Design review of the part built by this model. Coordinates are the model's own, in mm. Give positions to 0.01 mm unless a question says otherwise; leave off trailing zeros. Loops run counter-clockwise (first coordinate to the right, second up) from the corner with the lowest first, then second, coordinate; pieces in that order, holes last. Notation, with made-up numbers: M -14.75,1.25 L 24.25,1.25 A31 cw 24.25,37.25 Z; hole C 29,5 d10. An arc over 180 degrees is marked long. Use one line per item in the form item = value. Start each with the question number.
from build123d import *

# Parameters (mm, degrees)
F1_DEPTH = 25.4


with BuildPart() as f1:
    # F0 (on Top) → F1 (new body)
    with BuildSketch(Plane.XY):
        with BuildLine():
            Line((34.00621, -112.865897), (295.52461, -65.317097))
            Line((295.52461, -65.317097), (295.52461, 99.782903))
            Line((295.52461, 99.782903), (181.341427, 165.706594))
            Line((181.341427, 165.706594), (-34.67539, 87.082903))
            Line((-34.67539, 87.082903), (-34.67539, -65.317097))
            ThreePointArc((-34.67539, -65.317097), (-19.796415, -101.238122), (16.12461, -116.117097))
            Line((16.12461, -116.117097), (34.00621, -112.865897))
        make_face()
        with BuildLine():
            ThreePointArc((16.12461, -116.117097), (25.21199, -115.297689), (34.00621, -112.865897))
            Line((34.00621, -112.865897), (16.12461, -116.117097))
        make_face()
    extrude(amount=F1_DEPTH)


solid = f1.part
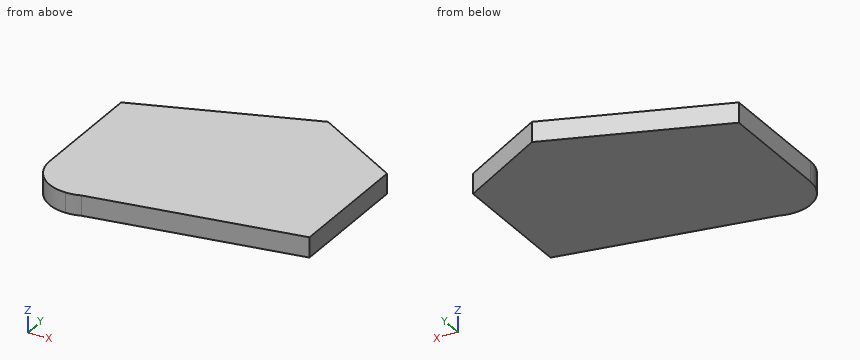
Q1. Take a section at C-C on x = 188. Give the boundary of the cut face in (y, z).
Q2. Wall thickness on probe 1 along Y at (x, z) = (136, 10.5); probe 2 along Y at (x, z) = (103, 23): over which ranges is each line inside the solid? List them lowest first.
Q3. Take a section at B-B on y = -71.5. Give the boundary of the cut face in (x, z), plus the area to 3 significant figures.
Q4. Take a section at A-A on z = 10. Give the boundary of the cut face in (x, y).
Q5. Clearance check with flat-ended pins moving along their axes: pin 1 Ø1 at (x, y) = (153.5, -63.5) entering from -Z; pin 2 Ø1.5 at (x, z) = (255, 6) entering from -Y; pin 3 Ø12 at (x, z) = (225, 5.5) entering from +Y; pin 4 Ø12 at (x, z) = (89.5, 3) entering from -Y. State where each tip first meets the part, or that it passes through.
Response values:
q1.outline = M -84.87,0 L 161.86,0 L 161.86,25.4 L -84.87,25.4 Z
q2.probe_1 = -94.32 to 149.2
q2.probe_2 = -100.32 to 137.19
q3.outline = M -34.3,0 L 261.52,0 L 261.52,25.4 L -34.3,25.4 Z
q3.area = 7,510 mm^2
q4.outline = M -34.68,-65.32 A50.8 ccw 16.12,-116.12 A50.8 ccw 34.01,-112.87 L 295.52,-65.32 L 295.52,99.78 L 181.34,165.71 L -34.68,87.08 Z
q5.pin_1 = 0
q5.pin_2 = -72.82
q5.pin_3 = 143.96
q5.pin_4 = -103.87
